Geometry check sheet. Reference: the model listing, model coordinates, mm. Round coordinates to 2 decimals unless told otherwise and drop trailing zeros. Loops run counter-clockwise (first coordinate to the right, second up) from the corner with the lowest first, then second, coordinate; pieces in that order, holes last. Notation, with made-up numbers: (-31, 68) - (-10, 68) arc R31 cw to (-10, 98) - close; hole circle Ø1 at (61, 51). An arc over 180 degrees is marked (long way). Answer as CSV lines item,"result". Start each with the question number.
1) Cross-section at B-B on y = 0. Record the boundary of the cut face in (x, z).
2) Depth check by flat-ended pin: P1, Ø4, axis at x = 28.28, y = 28.28, coming from the -Z side; P2, Ø5, axis at x = -28.28, y = 28.28, coming from the -Z side; P3, Ø1, axis at x = 12.5, z = 1, coming from the -Y side. Enter the tip coordinate at first touch or a pass-through.
3) Cross-section at A-A on x = 0. Record the boundary of the cut face in (y, z), and give its area (3 significant figures).
4) Cross-section at C-C on z = 1.2. State how many separate pieces and enclosed holes the cut face has, and give its area (3 significant figures).
5) Thickness scan on line 1 along Y through (x, z) = (0, 2.4); line 2 along Y through (x, z) = (28, 0.9); line 3 along Y through (x, z) = (14.5, 0.95). Record the ranges inside material, lowest first.
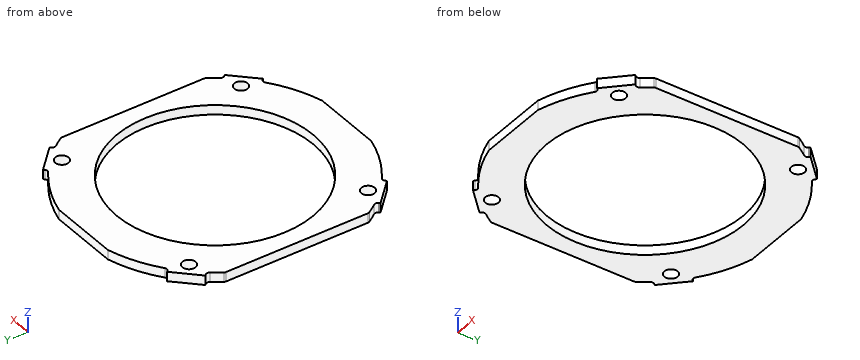
from build123d import *

# Parameters (mm, degrees)
SKETCH001_R   = 31
SKETCH001_R_2 = 2.1
PAD_DEPTH     = 3
FILLET_R      = 1


with BuildPart() as part:
    # Sketch001 → Pad (new body)
    with BuildSketch(Plane.XY):
        with BuildLine():
            Line((-36.5, 22.732136), (-36.5, -22.732136))
            ThreePointArc((-36.5, -22.732136), (-35.172415, -24.736637), (-33.734872, -26.663804))
            Line((-33.734872, -26.663804), (-34.718943, -27.647875))
            Line((-34.718943, -27.647875), (-27.647875, -34.718943))
            Line((-27.647875, -34.718943), (-26.663804, -33.734872))
            ThreePointArc((-26.663804, -33.734872), (-19.180875, -38.484985), (-10.883014, -41.6))
            Line((-10.883014, -41.6), (10.883014, -41.6))
            ThreePointArc((10.883014, -41.6), (19.180875, -38.484985), (26.663804, -33.734872))
            Line((26.663804, -33.734872), (27.647875, -34.718943))
            Line((27.647875, -34.718943), (34.718943, -27.647875))
            Line((34.718943, -27.647875), (33.734872, -26.663804))
            ThreePointArc((33.734872, -26.663804), (35.172415, -24.736637), (36.5, -22.732136))
            Line((36.5, -22.732136), (36.5, 22.732136))
            ThreePointArc((36.5, 22.732136), (35.172415, 24.736637), (33.734872, 26.663804))
            Line((34.718943, 27.647875), (33.734872, 26.663804))
            Line((27.647875, 34.718943), (34.718943, 27.647875))
            Line((26.663804, 33.734872), (27.647875, 34.718943))
            ThreePointArc((26.663804, 33.734872), (19.180875, 38.484985), (10.883014, 41.6))
            Line((10.883014, 41.6), (-10.883014, 41.6))
            ThreePointArc((-10.883014, 41.6), (-19.180875, 38.484985), (-26.663804, 33.734872))
            Line((-27.647875, 34.718943), (-26.663804, 33.734872))
            Line((-34.718943, 27.647875), (-27.647875, 34.718943))
            Line((-33.734872, 26.663804), (-34.718943, 27.647875))
            ThreePointArc((-33.734872, 26.663804), (-35.172415, 24.736637), (-36.5, 22.732136))
        make_face()
        Circle(SKETCH001_R, mode=Mode.SUBTRACT)
        with Locations((-28.284271, 28.284271)):
            Circle(SKETCH001_R_2, mode=Mode.SUBTRACT)
        with Locations((28.284271, 28.284271)):
            Circle(SKETCH001_R_2, mode=Mode.SUBTRACT)
        with Locations((28.284271, -28.284271)):
            Circle(SKETCH001_R_2, mode=Mode.SUBTRACT)
        with Locations((-28.284271, -28.284271)):
            Circle(SKETCH001_R_2, mode=Mode.SUBTRACT)
    extrude(amount=PAD_DEPTH)

    # Fillet
    fillet_edges = [part.edges().sort_by_distance(p)[0] for p in [
        (-26.663804, 33.734872, 1.5),
        (26.663804, 33.734872, 1.5),
        (33.734872, 26.663804, 1.5),
        (26.663804, -33.734872, 1.5),
        (33.734872, -26.663804, 1.5),
        (-26.663804, -33.734872, 1.5),
        (-33.734872, -26.663804, 1.5),
        (-33.734872, 26.663804, 1.5),
        (-36.5, -22.732136, 1.5),
        (-36.5, 22.732136, 1.5),
        (36.5, 22.732136, 1.5),
        (36.5, -22.732136, 1.5),
    ]]
    fillet(fillet_edges, radius=FILLET_R)


solid = part.part
Answer block:
1,outline,"(-36.5, 0) - (-31, 0) - (-31, 3) - (-36.5, 3) - close; (31, 0) - (36.5, 0) - (36.5, 3) - (31, 3) - close"
2,P1,"passes through"
2,P2,"stops at z = 0"
2,P3,"stops at y = -41.29"
3,outline,"(-41.6, 0) - (-31, 0) - (-31, 3) - (-41.6, 3) - close; (31, 0) - (41.6, 0) - (41.6, 3) - (31, 3) - close"
3,area,"63.6 mm^2"
4,separate pieces,"1"
4,enclosed holes,"5"
4,area,"2,340 mm^2"
5,line 1,"y = -41.6 to -31, 31 to 41.6"
5,line 2,"y = -34.37 to -30.36, -26.2 to -13.3, 13.3 to 26.2, 30.36 to 34.37"
5,line 3,"y = -40.48 to -27.4, 27.4 to 40.48"
